Build history of the part. All positions in model axes, mm. Round coordinates to 2 decimals unless told otherwise and drop trailing zeros. Order: outer loops, then holes, each group sorted by start corner. A loop starts at its lowest first (then second) coordinate and runs counter-clockwise, first axis right, second up. Notation, with made-up numbers: (51, -37) -> (58, -37) arc R15 ccw to (58, -32) -> close; hole circle Ø10 at (89, -9). An arc over 180 degrees is marked (long way). Answer as a JSON object with one key per item and string values.
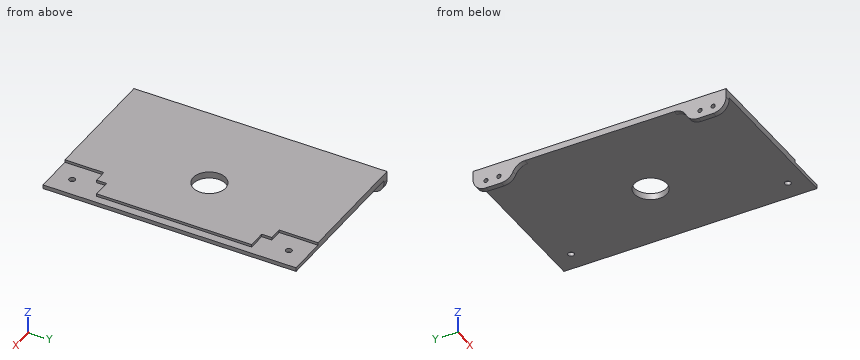
from build123d import *

# Parameters (mm, degrees)
CROQUIS1_W                  = 248.76
CROQUIS1_H                  = 195
SALIENTE_EXTRUIR1_DEPTH     = 5
CROQUIS2_W                  = 48
CROQUIS2_H                  = 30
CROQUIS2_W_2                = 30
CORTAR_EXTRUIR1_DEPTH       = 2
CROQUIS3_R                  = 2.375
CORTAR_EXTRUIR2_DEPTH       = 10
CROQUIS4_R                  = 40
SALIENTE_EXTRUIR2_DEPTH     = 206
CROQUIS5_R                  = 12.5
CORTAR_EXTRUIR3_DEPTH       = 10
CROQUIS12_W                 = 12
CROQUIS12_H                 = 30
SALIENTE_EXTRUIR3_DEPTH     = 4
REDONDEO1_R                 = 10
REDONDEO2_R                 = 10
REDONDEO3_R                 = 10
CORTAR_EXTRUIR5_DEPTH       = 262.677217236
CORTAR_EXTRUIR5_DEPTH_BACK  = 262.677217236
CROQUIS13_R                 = 1.625
CORTAR_EXTRUIR7_DEPTH       = 2
CROQUIS16_R                 = 1.75
CORTAR_EXTRUIR9_DEPTH       = 20
CORTAR_EXTRUIR16_DEPTH      = 264.206105047
CORTAR_EXTRUIR16_DEPTH_BACK = 264.206105047
CROQUIS14_W                 = 124.38
CROQUIS14_H                 = 195


with BuildPart() as part:
    # Croquis1 → Saliente-Extruir1 (new body)
    with BuildSketch(Plane.XY):
        with Locations((7.088293187, 0.26268)):
            Rectangle(CROQUIS1_W, CROQUIS1_H)
    extrude(amount=SALIENTE_EXTRUIR1_DEPTH)

    # Croquis2 → Cortar-Extruir1 (cut)
    with BuildSketch(Plane.XY.offset(5)):
        with Locations((-93.291706813, -82.23732)):
            Rectangle(CROQUIS2_W, CROQUIS2_H)
        with Locations((116.468293187, 82.76268)):
            Rectangle(CROQUIS2_W_2, CROQUIS2_H)
        with Locations((116.468293187, -82.23732)):
            Rectangle(CROQUIS2_W_2, CROQUIS2_H)
        with Locations((-93.291706813, 82.76268)):
            Rectangle(CROQUIS2_W, CROQUIS2_H)
    extrude(amount=-CORTAR_EXTRUIR1_DEPTH, mode=Mode.SUBTRACT)

    # Croquis3 → Cortar-Extruir2 (cut)
    with BuildSketch(Plane.XY.offset(5)):
        with Locations((-93.291706813, 83.76268)):
            Circle(CROQUIS3_R)
        with Locations((-93.291706813, -83.23732)):
            Circle(CROQUIS3_R)
        with Locations((116.468293187, 83.76268)):
            Circle(CROQUIS3_R)
        with Locations((116.468293187, -83.23732)):
            Circle(CROQUIS3_R)
    extrude(amount=-CORTAR_EXTRUIR2_DEPTH, mode=Mode.SUBTRACT)

    # Croquis4 → Saliente-Extruir2 (add)
    with BuildSketch(Plane(origin=(0, 0, 0), x_dir=(-1, 0, 0), z_dir=(0, 0, -1))):
        with Locations(Location((55.101706813, 0.26268, 0), (0, 0, 180))):
            Circle(CROQUIS4_R)
    extrude(amount=SALIENTE_EXTRUIR2_DEPTH)

    # Croquis5 → Cortar-Extruir3 (cut)
    with BuildSketch(Plane(origin=(0, 0, 0), x_dir=(-1, 0, 0), z_dir=(0, 0, -1))):
        with Locations((-76.968293187, 0.26268)):
            Circle(CROQUIS5_R)
    extrude(amount=-CORTAR_EXTRUIR3_DEPTH, mode=Mode.SUBTRACT)

    # Croquis12 → Saliente-Extruir3 (add, symmetric)
    with BuildSketch(Plane(origin=(7.088293187, 0, 0), x_dir=(0, 0, -1), z_dir=(1, 0, 0))):
        with Locations((6, 82.76268)):
            Rectangle(CROQUIS12_W, CROQUIS12_H)
        with Locations((6, -82.23732)):
            Rectangle(CROQUIS12_W, CROQUIS12_H)
    extrude(amount=SALIENTE_EXTRUIR3_DEPTH, both=True)

    # Redondeo1
    redondeo1_edges = [part.edges().sort_by_distance(p)[0] for p in [
        (7.088293187, 67.76268, 0),
        (7.088293187, -67.23732, 0),
    ]]
    fillet(redondeo1_edges, radius=REDONDEO1_R)

    # Redondeo2
    redondeo2_edges = [part.edges().sort_by_distance(p)[0] for p in [
        (7.088293187, 67.76268, -12),
        (7.088293187, -67.23732, -12),
    ]]
    fillet(redondeo2_edges, radius=REDONDEO2_R)

    # Redondeo3
    redondeo3_edges = [part.edges().sort_by_distance(p)[0] for p in [
        (7.088293187, 97.76268, -12),
        (7.088293187, -97.23732, -12),
    ]]
    fillet(redondeo3_edges, radius=REDONDEO3_R)

    # Croquis13 → Cortar-Extruir5 (cut, two sides: drawn at the far end of the back side and taken through both)
    with BuildSketch(Plane(origin=(11.088293187, 0, 0), x_dir=(0, 0, -1), z_dir=(1, 0, 0)).offset(-CORTAR_EXTRUIR5_DEPTH_BACK)):
        with Locations(Location((6, 87.76268, 0), (0, 0, 90))):
            Circle(CROQUIS13_R)
        with Locations(Location((6, 77.76268, 0), (0, 0, 90))):
            Circle(CROQUIS13_R)
        with Locations(Location((6, -77.23732, 0), (0, 0, 90))):
            Circle(CROQUIS13_R)
        with Locations(Location((6, -87.23732, 0), (0, 0, 90))):
            Circle(CROQUIS13_R)
    extrude(amount=CORTAR_EXTRUIR5_DEPTH + CORTAR_EXTRUIR5_DEPTH_BACK, mode=Mode.SUBTRACT)

    # Croquis15 → Cortar-Extruir7 (cut)
    with BuildSketch(Plane.XY.offset(5)):
        Polygon((111.468293187, 67.76268), (131.468293187, 67.76268), (131.468293187, -67.23732), (111.468293187, -67.23732), (111.468293187, -59.48732), (125.218293187, -59.48732), (125.218293187, 60.01268), (111.468293187, 60.01268), align=None)
    extrude(amount=-CORTAR_EXTRUIR7_DEPTH, mode=Mode.SUBTRACT)

    # Croquis16 → Cortar-Extruir9 (cut)
    with BuildSketch(Plane.XY.offset(5)):
        with Locations((-55.101706813, 20.26268)):
            Circle(CROQUIS16_R)
        with Locations((-35.101706813, 0.26268)):
            Circle(CROQUIS16_R)
        with Locations((-55.101706813, -19.73732)):
            Circle(CROQUIS16_R)
        with Locations((-75.101706813, 0.26268)):
            Circle(CROQUIS16_R)
    extrude(amount=-CORTAR_EXTRUIR9_DEPTH, mode=Mode.SUBTRACT)

    # Croquis14 → Cortar-Extruir16 (cut, two sides: drawn at the far end of the back side and taken through both)
    with BuildSketch(Plane(origin=(0, 0, 0), x_dir=(-1, 0, 0), z_dir=(0, 0, -1)).offset(-CORTAR_EXTRUIR16_DEPTH_BACK)):
        with Locations((55.101706813, 0.26268)):
            Rectangle(CROQUIS14_W, CROQUIS14_H)
    extrude(amount=CORTAR_EXTRUIR16_DEPTH + CORTAR_EXTRUIR16_DEPTH_BACK, mode=Mode.SUBTRACT)


solid = part.part
1) Cut at C-C, the plane x = 105.5. Give the cut face in (y, z), plus the area to 3 significant figures.
Checked values:
{"outline": "(-97.24, 0) -> (97.76, 0) -> (97.76, 3) -> (67.76, 3) -> (67.76, 5) -> (-67.24, 5) -> (-67.24, 3) -> (-97.24, 3) -> close", "area": "855 mm²"}
2) Probe L1, parallel to Z at x = 59, y = -23; L2, parallel to X at y = -64.5, z = -0.5. List the from-to ranges inside material, lowest first. Write a range as from..to.
Checked values:
{"L1": "z = 0..5", "L2": "x = 7.09..11.09"}
3) Cut at A-A, the plane x = 83. Give the cut face in (y, z), plus the area to 3 significant figures.
Checked values:
{"outline": "(-97.24, 0) -> (-10.69, 0) -> (-10.69, 5) -> (-97.24, 5) -> close; (11.21, 0) -> (97.76, 0) -> (97.76, 5) -> (11.21, 5) -> close", "area": "866 mm²"}
4) Cut at B-B, the plane y = -7.5. Give the cut face in (x, z), plus the area to 3 significant figures.
Checked values:
{"outline": "(7.09, 0) -> (67.17, 0) -> (67.17, 5) -> (7.09, 5) -> close; (86.77, 0) -> (131.47, 0) -> (131.47, 3) -> (125.22, 3) -> (125.22, 5) -> (86.77, 5) -> close", "area": "511 mm²"}
5) Cut at D-D, the plane x = 22.5. Give the cut face in (y, z).
Checked values:
{"outline": "(-97.24, 0) -> (97.76, 0) -> (97.76, 5) -> (-97.24, 5) -> close"}
6) Flat gauge pins, fed straight in: pin 1 Ø7.5 at (x, y) = (116.47, 83.76) entering from +Z; pin 2 Ø8 at (x, y) = (84.5, 22) entering from -Z; pin 3 Ø3.5 at (y, z) = (-78.5, -5) entering from +X; pin 4 Ø1.5 at (y, z) = (39, -2.5) entering from -X. Where does each tip first touch, or does it go through?
Checked values:
{"pin 1": "stops at z = 3", "pin 2": "stops at z = 0", "pin 3": "stops at x = 11.09", "pin 4": "passes through"}
